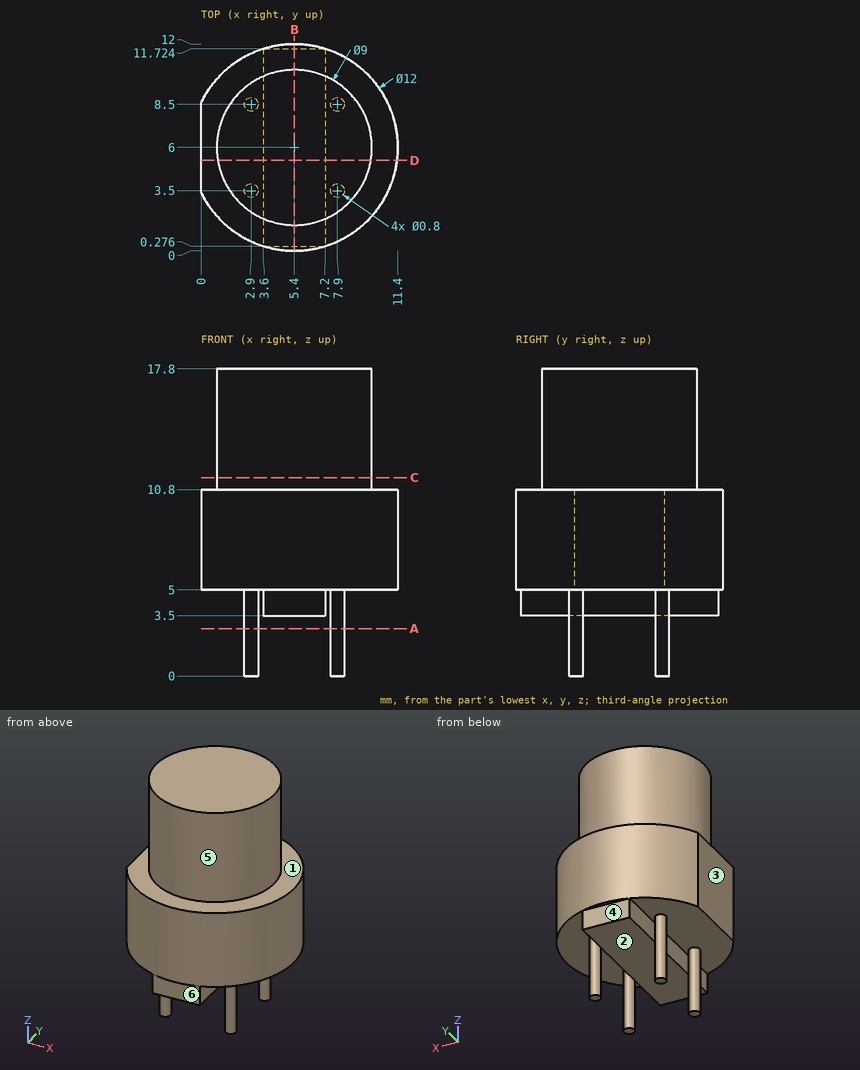
Geometry check sheet. Reference: drawing and pictorial views, mm from the part's lowest x, y, z. A direction names the side the tool comes from. Round coordinates to 2 decimals unless told otherwise and drop trailing zeros. Write each loop counter-clockwise with the first axis right and the second up, starting at its lowest first coordinate (ties: lowest second). Pieces come first, ordered by that corner, then holes.
1. Draft check along X on the marked faces 1, 2 and 3. Enter one of: +X half, -X half, draft (parallel to the pull), parting line (faces both ways), or undercut.
2. Section check A-A on z = 2.75. Enter the section's corners in (x, y).
3. Section check C-C on z = 11.5. Enter the section's corners in (x, y).
4. Access from +Z, -Z, +X, -X, +Y, -Y to the whole of each face (thin tool, end or side, straight path). Record for the marked faces 4, 5 and 6.
5. Scan lines: L1, parallel to Z at x = 5, y = 2.25; L2, parallel to Z at x = 3.5, y = 5.5; L3, parallel to Y at x = 4.5, z = 3.75. Record each from-to range of solid material in increasing order.
6. Section check B-B on x = 5.4. Enter the section's corners in (y, z).
7. Gauge pin test, flat ends, axial feed: P1, Ø1.5, axis at x = 10, y = 10.5, coming from the +Z side; P2, Ø1.6, axis at y = 7, z = 4, coming from the +X side; P3, Ø6, axis at y = 2.5, z = 11, coming from the +X side; P4, Ø3, axis at x = 3, y = 2, coming from the +Z side. Record the tip position at first contact, or that the pin passes through.
8. Section check D-D on y = 5.25. Enter the section's corners in (x, z), plus the area to 3 significant figures.
Answer:
1. face 1: draft
1. face 2: undercut
1. face 3: -X half
2. outline: circle Ø0.8 at (2.9, 3.5); circle Ø0.8 at (2.9, 8.5); circle Ø0.8 at (7.9, 3.5); circle Ø0.8 at (7.9, 8.5)
3. outline: circle Ø9 at (5.4, 6)
4. face 4: -Z, +X, -X, +Y
4. face 5: +Z
4. face 6: -Z, +X, -X, -Y
5. L1: z = 3.5 to 17.8
5. L2: z = 5 to 17.8
5. L3: y = 0.28 to 11.72
6. outline: (0, 5) - (0.28, 5) - (0.28, 3.5) - (11.72, 3.5) - (11.72, 5) - (12, 5) - (12, 10.8) - (10.5, 10.8) - (10.5, 17.8) - (1.5, 17.8) - (1.5, 10.8) - (0, 10.8) - close
7. P1: stops at z = 10.8
7. P2: stops at x = 7.2
7. P3: stops at x = 11.38
7. P4: stops at z = 17.8
8. outline: (0, 5) - (3.6, 5) - (3.6, 3.5) - (7.2, 3.5) - (7.2, 5) - (11.35, 5) - (11.35, 10.8) - (9.84, 10.8) - (9.84, 17.8) - (0.96, 17.8) - (0.96, 10.8) - (0, 10.8) - close
8. area: 133 mm2
